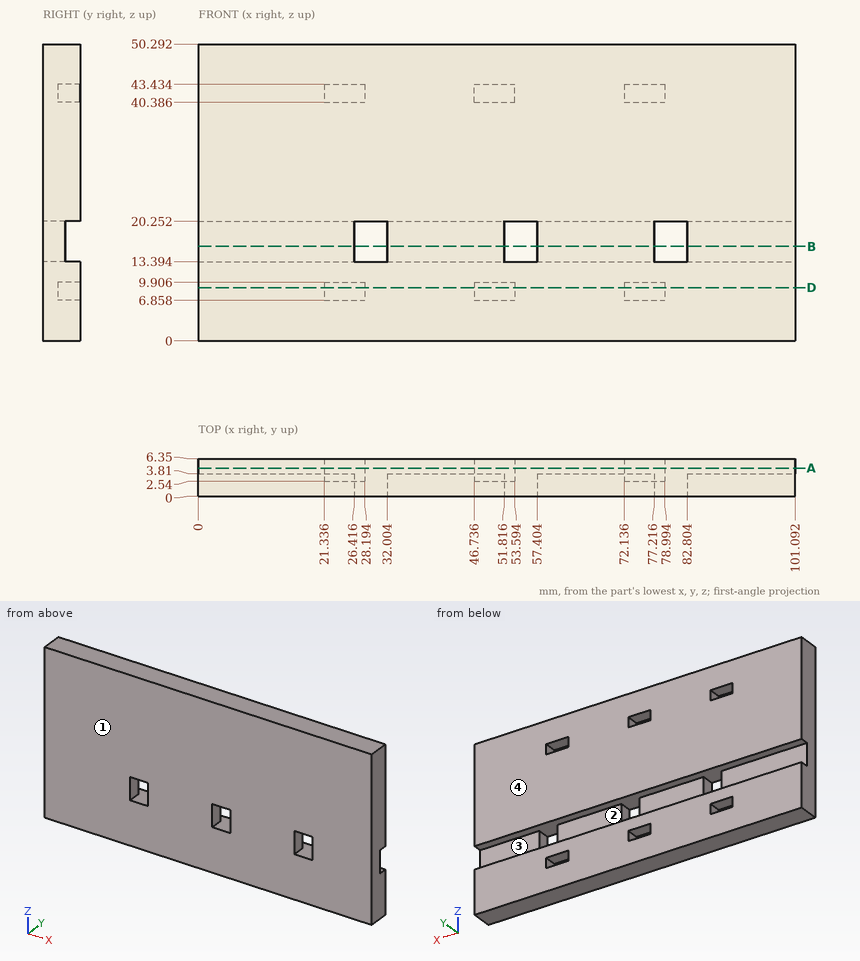
Check sheet for the drawn part. Datum: minimum x, y, z corner. Units: mm. A direction names the side the tool comes from. Round coordinates to 2 decimals unless told otherwise and drop trailing zeros. Write each loop counter-clockwise with the first axis right and the second up, starting at its lowest first coordinate (ties: lowest second). Pieces come first, ordered by that corner, then holes. Notation, with made-up numbers: (-2, 66) -> (5, 66) arc R22 ccw to (5, 98) -> close; hole circle Ø2 at (82, -31.5). An arc over 180 degrees is marked (long way). Put each result on its own line as item: value.
(1) Sectioned sample at B-B (z = 16). Enter the section's corners in (x, y), plus the area to 3 significant figures.
Values found:
outline: (0, 0) -> (26.42, 0) -> (26.42, 3.81) -> (0, 3.81) -> close; (32, 0) -> (51.82, 0) -> (51.82, 3.81) -> (32, 3.81) -> close; (57.4, 0) -> (77.22, 0) -> (77.22, 3.81) -> (57.4, 3.81) -> close; (82.8, 0) -> (101.09, 0) -> (101.09, 3.81) -> (82.8, 3.81) -> close
area: 321 mm^2
(2) Material ranges on line 1 (Z direction, x = 76, y = 4.5) (1 decimal); line 2 (X direction, y = 0.5, z = 16.5); line 3 (Z direction, x = 17, y = 4.75) (1 decimal), recorded low to high.
Values found:
line 1: z = 0 to 6.9, 9.9 to 13.4, 20.3 to 40.4, 43.4 to 50.3
line 2: x = 0 to 26.42, 32 to 51.82, 57.4 to 77.22, 82.8 to 101.09
line 3: z = 0 to 13.4, 20.3 to 50.3
(3) Sectioned sample at D-D (z = 9). Enter the section's corners in (x, y).
Values found:
outline: (0, 0) -> (101.09, 0) -> (101.09, 6.35) -> (78.99, 6.35) -> (78.99, 2.54) -> (72.14, 2.54) -> (72.14, 6.35) -> (53.59, 6.35) -> (53.59, 2.54) -> (46.74, 2.54) -> (46.74, 6.35) -> (28.19, 6.35) -> (28.19, 2.54) -> (21.34, 2.54) -> (21.34, 6.35) -> (0, 6.35) -> close
(4) Mould release check, pull along Z, two halves, no side actions. Record for the marked faces 1 and 2: released by +Z, released by -Z, zero draft, split by the parting line, or undercut.
Values found:
face 1: zero draft
face 2: undercut
(5) Sectioned sample at A-A (y = 4.75). Count the separate pieces of the cut face and the enclosed holes in it.
Values found:
separate pieces: 2
enclosed holes: 6
(6) Go/stop test with a flat-tipped pin: pin 1 Ø0.9 at (x, z) = (75.5, 42) entering from +Y. Record where the tip stops, or that it passes through.
Values found:
pin 1: stops at y = 2.54
(7) Tool access check on the marked faces 3 and 4. Record the directions out of +Z, -Z, +X, -X, +Y, -Y that give a thin tool (end or side, any length) a straight path to the whole face; none if there is none.
Values found:
face 3: +X, -X, +Y
face 4: +Z, -Z, +X, -X, +Y
